Read the model definition and answer for the solid it produces. Units are mm, in the model's axes. Give positions to 0.01 mm unless a question says otherwise; leave off trailing zeros. Loops run counter-clockwise (first coordinate to the right, second up) from the corner with the lowest first, then second, coordinate; pieces in that order, holes last. Notation, with made-up numbers: (-10, -4.5) - (12, -4.5) arc R22 cw to (12, 24.5) - close; hole circle Ø4 at (-25, 6). An arc over 180 degrees is marked (long way). Write item = value, one per line.
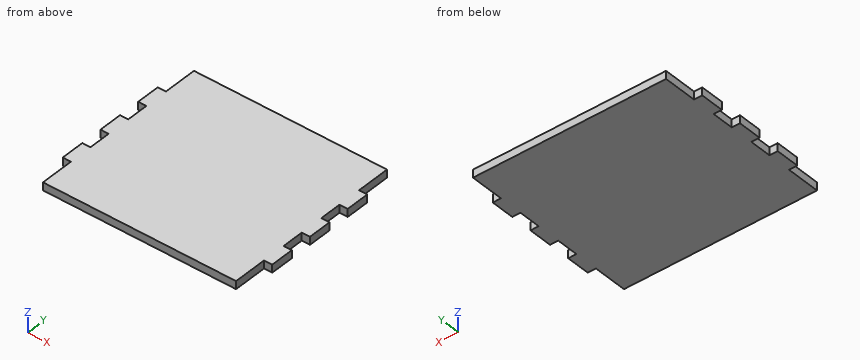
```python
from build123d import *

# Parameters (mm, degrees)
BOSS_EXTRUDE1_DEPTH = 3.175


with BuildPart() as part:
    # Sketch1 → Boss-Extrude1 (new body, symmetric)
    with BuildSketch(Plane.XY):
        Polygon((77.724, 73.025), (-77.724, 73.025), (-77.724, 45.974), (-84.328, 45.974), (-84.328, 27.051), (-77.724, 27.051), (-77.724, 9.4615), (-84.328, 9.4615), (-84.328, -9.4615), (-77.724, -9.4615), (-77.724, -27.051), (-84.328, -27.051), (-84.328, -45.974), (-77.724, -45.974), (-77.724, -73.025), (77.724, -73.025), (77.724, -45.974), (84.328, -45.974), (84.328, -27.051), (77.724, -27.051), (77.724, -9.4615), (84.328, -9.4615), (84.328, 9.4615), (77.724, 9.4615), (77.724, 27.051), (84.328, 27.051), (84.328, 45.974), (77.724, 45.974), align=None)
    extrude(amount=BOSS_EXTRUDE1_DEPTH, both=True)


solid = part.part
```
1) A cutting plane is placed at B-B on y = -50.5. Determine the outline of the cut face in (x, z) (3 decimals), then the cut area to 3 significant figures.
Output:
outline = (-77.724, -3.175) - (77.724, -3.175) - (77.724, 3.175) - (-77.724, 3.175) - close
area = 987 mm²
2) A cutting plane is placed at A-A on z = 0.5. Determine the outline of the cut face in (x, y) (1 decimal).
Output:
outline = (-84.3, -46) - (-77.7, -46) - (-77.7, -73) - (77.7, -73) - (77.7, -46) - (84.3, -46) - (84.3, -27.1) - (77.7, -27.1) - (77.7, -9.5) - (84.3, -9.5) - (84.3, 9.5) - (77.7, 9.5) - (77.7, 27.1) - (84.3, 27.1) - (84.3, 46) - (77.7, 46) - (77.7, 73) - (-77.7, 73) - (-77.7, 46) - (-84.3, 46) - (-84.3, 27.1) - (-77.7, 27.1) - (-77.7, 9.5) - (-84.3, 9.5) - (-84.3, -9.5) - (-77.7, -9.5) - (-77.7, -27.1) - (-84.3, -27.1) - close
3) Each of these flat-tipped pins is pushed along its axis until it touches: P1, Ø1.9, axis at x = 79.5, z = -0.5, coming from the +Y side; P2, Ø2, axis at y = 55, z = 1.5, coming from the -X side; P3, Ø1.9, axis at x = 82.5, z = 1, coming from the -Y side. Where does it stop, or does it pass through?
Output:
P1 = 45.97
P2 = -77.72
P3 = -45.97
4) Find the intervals of material crossed by probe 1 along X at (y, z) = (11.5, -0.25), in increasing order.
Output:
probe_1 = -77.72 to 77.72
